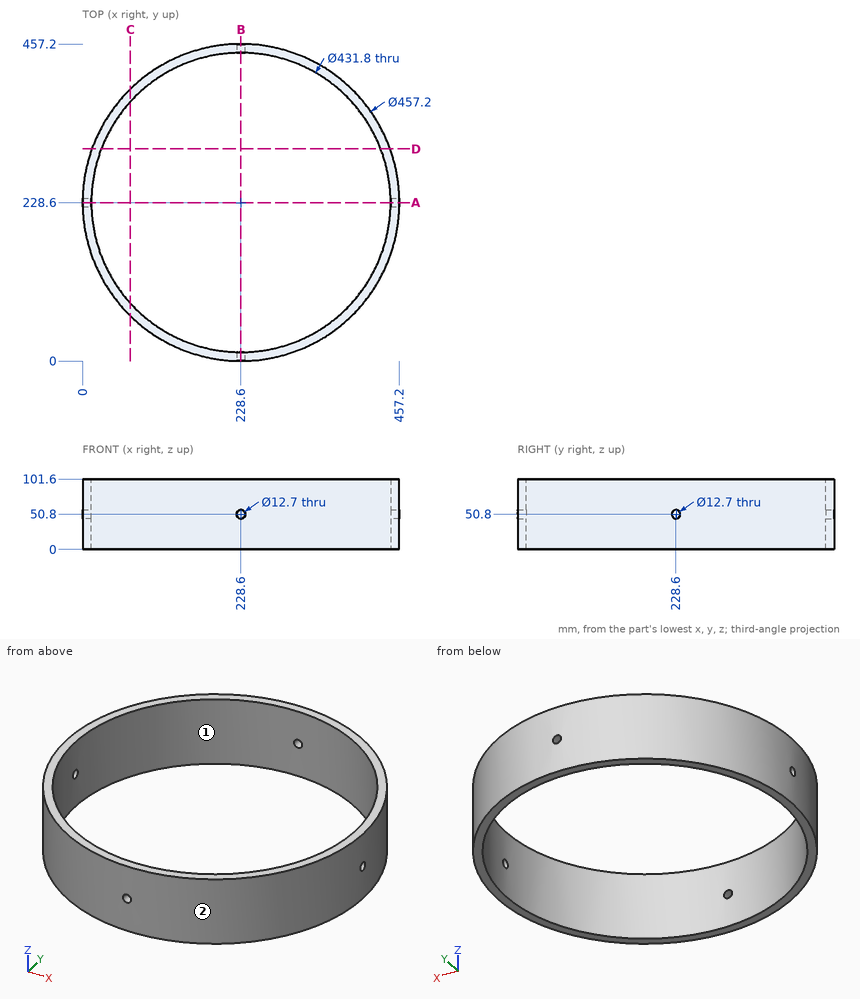
Study the drawing (mm; zero at the part's minimum x, y, z) and answer. Give positions to 0.01 mm unless a question says otherwise; leave off trailing zeros. Write each loop counter-clockwise with the first axis right and the second up, starting at its lowest first coordinate (ties: lowest second). Pieces come first, ordered by that corner, then holes. Notation, with made-up numbers: (41.5, 56.5) -> (46.5, 56.5) arc R19 ccw to (46.5, 91.5) -> close; hole circle Ø11 at (-14.75, 20.25). An arc over 180 degrees is marked (long way). Answer as a JSON object with one key per item and string values. Group by question number.
1) Consider L1, parallel to Z at x = 228.6, y = 454.5; L2, parallel to X at y = 234.5, z = 31.5; L3, parallel to Y at x = 228, z = 17.5. Determine where each line is inside the solid, lowest interval first. Write a range as from..to.
2) Find section D-D (y = 306). Write down the section's boundary in (x, z).
3) Each of these flat-tipped pins is pushed along its axis until it touches: P1, Ø6, axis at x = 257.5, z = 11, coming from the +Y side; P2, Ø8, axis at y = 111.5, z = 69, coming from the +X side; P3, Ø7.5, axis at x = 228.6, z = 50.8, coming from the +Y side; P4, Ø4, axis at x = 160.5, z = 32.5, coming from the +Y side (3 decimals). Where does it stop, or does it pass through?
4) Find section C-C (x = 69). Write down the section's boundary in (y, z), and give its area (3 significant figures).
5) The mould has two halves that part along Y. Classify the marked faces 1 and 2: +Y half, -Y half, draft (parallel to the pull), parting line (faces both ways), or undercut.
6) Find section A-A (y = 228.6). Write down the section's boundary in (x, z).
Values follow:
{
 "1": {"L1": "z = 0..44.45, 57.15..101.6", "L2": "x = 0.08..12.78, 444.42..457.12", "L3": "y = 0..12.7, 444.5..457.2"},
 "2": {"outline": "(13.5, 0) -> (27.05, 0) -> (27.05, 101.6) -> (13.5, 101.6) -> close; (430.15, 0) -> (443.7, 0) -> (443.7, 101.6) -> (430.15, 101.6) -> close"},
 "3": {"P1": "stops at y = 455.73", "P2": "stops at x = 427.26", "P3": "passes through", "P4": "stops at y = 447.435"},
 "4": {"outline": "(64.94, 0) -> (83.2, 0) -> (83.2, 101.6) -> (64.94, 101.6) -> close; (374, 0) -> (392.26, 0) -> (392.26, 101.6) -> (374, 101.6) -> close", "area": "3,710 mm2"},
 "5": {"face 1": "undercut", "face 2": "parting line"},
 "6": {"outline": "(0, 0) -> (12.7, 0) -> (12.7, 44.45) -> (0, 44.45) -> close; (0, 57.15) -> (12.7, 57.15) -> (12.7, 101.6) -> (0, 101.6) -> close; (444.5, 0) -> (457.2, 0) -> (457.2, 44.45) -> (444.5, 44.45) -> close; (444.5, 57.15) -> (457.2, 57.15) -> (457.2, 101.6) -> (444.5, 101.6) -> close"}
}
